from build123d import *

# Parameters (mm, degrees)
F0_W      = 139.4050866365
F0_H      = 26.4991316944
F1_DEPTH  = 38.1
F3_DEPTH  = 26.162
F5_DEPTH  = 26.162
F6_R      = 20.3401801488
F6_R_2    = 18.3914355894
F7_DEPTH  = 26.5001316944
F8_W      = 78.8159519434
F8_H      = 50.5755208433
F9_DEPTH  = 50.8
F11_DEPTH = 63.3887604216
F12_W     = 29.0339104831
F12_H     = 34.9128932312
F13_DEPTH = 63.3887604216
F15_DEPTH = 22.86
F17_DEPTH = 26.416
F18_R     = 7.4156213221
F19_DEPTH = 146.9803799493


with BuildPart() as f1:
    # F0 (on Front) → F1 (new body, symmetric)
    with BuildSketch(Plane.XZ):
        Rectangle(F0_W, F0_H)
    extrude(amount=F1_DEPTH, both=True)

    # F2 (on face) → F3 (join)
    with BuildSketch(Plane.XY.offset(13.2495658472)):
        with BuildLine():
            Line((69.7025433183, 38.1), (69.7025433183, -38.1))
            ThreePointArc((69.7025433183, -38.1), (107.8025433183, 0), (69.7025433183, 38.1))
        make_face()
    extrude(amount=-F3_DEPTH)

    # F4 (on face) → F5 (join)
    with BuildSketch(Plane.XY.offset(13.2495658472)):
        with BuildLine():
            Line((-69.7025433183, -38.1), (-69.7025433183, 38.1))
            ThreePointArc((-69.7025433183, 38.1), (-107.8025433183, 0), (-69.7025433183, -38.1))
        make_face()
    extrude(amount=-F5_DEPTH)

    # F6 (on face) → F7 (cut, through all)
    with BuildSketch(Plane.XY.offset(13.2495658472)):
        with Locations((69.7025433183, 0)):
            Circle(F6_R)
        with Locations((-69.7025433183, 0)):
            Circle(F6_R_2)
    extrude(amount=-F7_DEPTH, mode=Mode.SUBTRACT)

    # F8 (on face) → F9 (join)
    with BuildSketch(Plane.XY.offset(13.2495658472)):
        Rectangle(F8_W, F8_H)
    extrude(amount=F9_DEPTH)

    # F10 (on face) → F11 (cut, through all)
    with BuildSketch(Plane(origin=(0, 25.2877604216, 0), x_dir=(-1, 0, 0), z_dir=(0, 1, 0))):
        with BuildLine():
            Line((12.7608366311, 29.136672616), (-16.2730738521, 29.136672616))
            ThreePointArc((-16.2730738521, 29.136672616), (-1.7561186105, 19.2027423091), (12.7608366311, 29.136672616))
        make_face()
    extrude(amount=-F11_DEPTH, mode=Mode.SUBTRACT)

    # F12 (on face) → F13 (cut, through all)
    with BuildSketch(Plane(origin=(0, 25.2877604216, 0), x_dir=(-1, 0, 0), z_dir=(0, 1, 0))):
        with Locations((-1.7561186105, 46.5931192316)):
            Rectangle(F12_W, F12_H)
    extrude(amount=-F13_DEPTH, mode=Mode.SUBTRACT)

    # F14 (on face) → F15 (join)
    with BuildSketch(Plane(origin=(16.2730738521, 0, 0), x_dir=(0, -1, 0), z_dir=(-1, 0, 0))):
        with BuildLine():
            Line((-25.2877604216, 64.0495658472), (25.2877604216, 64.0495658472))
            ThreePointArc((25.2877604216, 64.0495658472), (0, 89.3373262689), (-25.2877604216, 64.0495658472))
        make_face()
    extrude(amount=-F15_DEPTH)

    # F16 (on face) → F17 (join)
    with BuildSketch(Plane.YZ.offset(-12.7608366311)):
        with BuildLine():
            Line((-25.2877604216, 64.0495658472), (25.2877604216, 64.0495658472))
            ThreePointArc((25.2877604216, 64.0495658472), (0, 89.3373262689), (-25.2877604216, 64.0495658472))
        make_face()
    extrude(amount=-F17_DEPTH)

    # F18 (on face) → F19 (cut, through all)
    with BuildSketch(Plane(origin=(-39.1768366311, 0, 0), x_dir=(0, -1, 0), z_dir=(-1, 0, 0))):
        with Locations((0, 73.7898647785)):
            Circle(F18_R)
    extrude(amount=-F19_DEPTH, mode=Mode.SUBTRACT)


solid = f1.part
The listing builds one solid part. Answer for the finished solid, in the listing's coordinates (mm). A direction names the side the tool comes from. Give positions to 0.01 mm unless a question says otherwise; leave off trailing zeros. Loops run counter-clockwise (first coordinate to the right, second up) from the corner with the lowest first, then second, coordinate; pieces in that order, holes last.
Item 1: A cutting plane is placed at D-D (z = 7.5). Give the vertices of the cut face in (x, y).
Derived:
outline: (-69.7, -38.1) - (69.7, -38.1) arc R38.1 ccw to (69.7, 38.1) - (-69.7, 38.1) arc R38.1 ccw to start; hole circle Ø36.78 at (-69.7, 0); hole circle Ø40.68 at (69.7, 0)
Item 2: Each of these flat-tipped pins is pushed along its axis until it touches: pin 1 Ø2 at (y, z) = (0, 79) entering from -X; pin 2 Ø20 at (y, z) = (-6, 82.5) entering from +X; pin 3 Ø6 at (y, z) = (19.5, 67) entering from -X; pin 4 Ø15 at (x, z) = (-10.5, 30.5) entering from +Y. Where does it stop, or does it pass through?
Derived:
pin 1: passes through
pin 2: stops at x = 39.13
pin 3: stops at x = -39.41
pin 4: stops at y = 25.29
Item 3: A cutting plane is placed at A-A (z = 47.5). Give the vertices of the cut face in (x, y), then the cut area to 3 significant figures.
Derived:
outline: (-39.41, -25.29) - (-12.76, -25.29) - (-12.76, 25.29) - (-39.41, 25.29) - close; (16.27, -25.29) - (39.41, -25.29) - (39.41, 25.29) - (16.27, 25.29) - close
area: 2,520 mm2
Item 4: A cutting plane is placed at C-C (y = -10). Give the vertices of the cut face in (x, z).
Derived:
outline: (-106.47, -12.91) - (-85.14, -12.91) - (-85.14, 13.25) - (-106.47, 13.25) - close; (-54.27, -13.25) - (51.99, -13.25) - (51.99, 13.25) - (39.41, 13.25) - (39.41, 64.05) - (39.13, 64.05) - (39.13, 87.28) - (16.27, 87.28) - (16.27, 29.14) arc R15.57 cw to (-12.76, 29.14) - (-12.76, 87.28) - (-39.18, 87.28) - (-39.18, 64.05) - (-39.41, 64.05) - (-39.41, 13.25) - (-54.27, 13.25) - close; (87.41, -12.91) - (106.47, -12.91) - (106.47, 13.25) - (87.41, 13.25) - close
Item 5: Find the intervals of material crossed by line 1 along X through (y, z) = (0, 2.5); line 2 along Z through (x, y) = (21.25, 0); line 3 along X through (y, z) = (0.5, 43), in increasing order.
Derived:
line 1: x = -107.8 to -88.09, -51.31 to 49.36, 90.04 to 107.8
line 2: z = -13.25 to 66.37, 81.21 to 89.34
line 3: x = -39.41 to -12.76, 16.27 to 39.41
Item 6: A cutting plane is placed at B-B (y = 0). Give the number of separate pieces and of enclosed holes in the cut face, then the cut area to 3 significant figures.
Derived:
separate pieces: 5
enclosed holes: 0
area: 6,940 mm2
Item 7: A tool of negligible diameter and unlimited length cuts with its end or side. For faces 1 (the flat face through (93, 1, -12.912)), 2 (the flat face through (-18, 25.288, 38)), 3 (the flat face through (-12.761, 0, 60)), 4 (the flat face through (-18, -25.288, 38)), 5 (the flat face through (-39.408, 0, 38)), from which of +Z, -Z, +X, -X, +Y, -Y can it reach the whole face along a straight path? Write none if from no direction.
Derived:
face 1: -Z, +X, +Y, -Y
face 2: +Z, +X, -X, +Y
face 3: +Z, +Y, -Y
face 4: +Z, +X, -X, -Y
face 5: +Z, -X, +Y, -Y
Item 8: Determine the mould class of faces 6 (the flat face through (-1, -1, -13.25)), 7 (the cylindrical face through (27.54, 0.97, 81.14)), 8 (the cylindrical face through (-25.78, 0.56, 89.33)) for opening direction Z: +Z half, -Z half, draft (parallel to the pull), parting line (faces both ways), or undercut.
Derived:
face 6: -Z half
face 7: undercut
face 8: +Z half
